Source: CAD feature listing. Evaluate the final solid. Frame: model axes, mm. A direction names the side the tool comes from. Round coordinates to 2 decimals unless told otherwise and drop trailing zeros. Order: outer loops, then holes, each group sorted by start corner. A loop starts at its lowest first (then second) coordinate and runs counter-clockwise, first axis right, second up. Notation, with made-up numbers: (65, 87) -> (96, 87) arc R5 ccw to (96, 92) -> close; hole circle Ø10 at (75, 78.5). An arc over 180 degrees is marked (long way). Write item = value, one per line. Start each with the question number.
(1) Cut plane B-B on y = 23.5. Return the cut outline in (x, z), then the cut area to 3 significant figures.
(2) Contact query for flat-ended pins moving along their axis: pin 1 Ø0.6 at (y, z) = (9, 3) entering from -X; pin 2 Ø0.6 at (y, z) = (2, 3.5) entering from +X; pin 3 Ø1 at (x, z) = (-4.5, 4) entering from +Y. Output: stop coordinate, or through.
(3) Draft query along X for faces 4 (the face through (35.35, 34.37, 3.32)), 5 (the face through (-33.833, 2, 1)), 6 (the face through (2, 3, 4.318)). Return one class per face: released by +X, released by -X, zero draft, split by the parting line, or undercut.
(4) Ray query, line 1 (X direction, y = 16.5, z = 4); line 2 (Y direction, x = 30.5, z = 2.9); line 3 (Y direction, x = 36, z = 4.1). Return the intervals inside material, ascending.
(5) Reachability of faces 1 (the face through (-29.867, -28.879, 3.316)), 2 (the face through (-29.946, 34.286, 3.316)), 3 (the face through (3, 37, 2.286)) from +Z, -Z, +X, -X, +Y, -Y: full face, straight path, thin tool, end or side. Return the list, or none.
(6) Cut plane A-A on x = 23. Return the cut outline in (y, z).
from build123d import *

# Parameters (mm, degrees)
F0_W     = 73.152002
F0_H     = 71.018402
F1_DEPTH = 2.286
F3_W     = 68.275202
F3_H     = 66.141603
F4_DEPTH = 2.032
F5_R     = 5.08
F6_R     = 5.08
F7_R     = 5.08
F8_R     = 5.08


with BuildPart() as f1:
    # F0 (on Top) → F1 (new body)
    with BuildSketch(Plane.XY):
        with Locations((2.743201, 2.438402)):
            Rectangle(F0_W, F0_H)
    extrude(amount=F1_DEPTH)

    # F3 (on face) → F4 (join)
    with BuildSketch(Plane.XY.offset(2.286)):
        with Locations((2.743201, 2.7432)):
            Rectangle(F3_W, F3_H)
    extrude(amount=F4_DEPTH)

    # F5
    f5_edges = [f1.edges().sort_by_distance(p)[0] for p in [
        (36.880802, -30.327601, 3.302),
    ]]
    fillet(f5_edges, radius=F5_R)

    # F6
    f6_edges = [f1.edges().sort_by_distance(p)[0] for p in [
        (-31.3944, -30.327601, 3.302),
    ]]
    fillet(f6_edges, radius=F6_R)

    # F7
    f7_edges = [f1.edges().sort_by_distance(p)[0] for p in [
        (-31.3944, 35.814002, 3.302),
    ]]
    fillet(f7_edges, radius=F7_R)

    # F8
    f8_edges = [f1.edges().sort_by_distance(p)[0] for p in [
        (36.880802, 35.814002, 3.302),
    ]]
    fillet(f8_edges, radius=F8_R)


solid = f1.part
Evaluation:
q1.outline = (-33.83, 0) -> (39.32, 0) -> (39.32, 2.29) -> (36.88, 2.29) -> (36.88, 4.32) -> (-31.39, 4.32) -> (-31.39, 2.29) -> (-33.83, 2.29) -> close
q1.area = 306 mm^2
q2.pin_1 = -31.39
q2.pin_2 = 36.88
q2.pin_3 = 35.81
q3.face_4 = released by +X
q3.face_5 = released by -X
q3.face_6 = zero draft
q4.line_1 = -31.39 to 36.88
q4.line_2 = -30.33 to 35.81
q4.line_3 = -28.11 to 33.59
q5.face_1 = +Z, -X, -Y
q5.face_2 = +Z, -X, +Y
q5.face_3 = +Z
q6.outline = (-33.07, 0) -> (37.95, 0) -> (37.95, 2.29) -> (35.81, 2.29) -> (35.81, 4.32) -> (-30.33, 4.32) -> (-30.33, 2.29) -> (-33.07, 2.29) -> close
